from build123d import *

# Parameters (mm, degrees)
SKETCH_1_W      = 53
SKETCH_1_H      = 53
EXTRUDE_1_DEPTH = 10
SKETCH_2_R      = 3


with BuildPart() as part:
    # 草图1 → 凸台-拉伸1 (new body)
    with BuildSketch(Plane.XY):
        with Locations((26.5, 26.5)):
            Rectangle(SKETCH_1_W, SKETCH_1_H)
    extrude(amount=EXTRUDE_1_DEPTH)

    # 扫描1: sweep along a path in 草图4
    with BuildLine(Plane(origin=(0, 0, 0), x_dir=(0, 0, -1), z_dir=(1, 0, 0))) as sweep_1_path:
        Line((-5, 0), (-5, -17))
        Line((-5, -17), (191, -17))
    # 草图2 → 扫描1 (sweep)
    with BuildSketch(Plane(origin=(0, 0, 0), x_dir=(1, 0, 0), z_dir=(0, 1, 0))):
        with Locations((12, -5)):
            Circle(SKETCH_2_R)
    sweep(path=sweep_1_path.line, transition=Transition.RIGHT)


solid = part.part
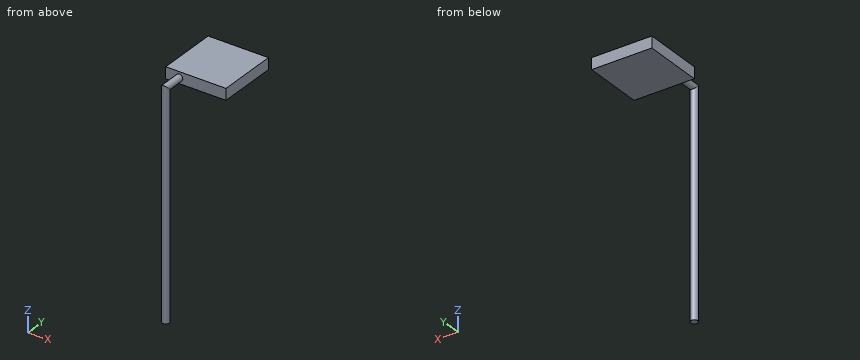
Verification items for the finished model (mm, model axes). Coordinates: 2 decimals unless noted, no trailing zeros. Loops run counter-clockwise (first coordinate to the right, second up) from the corner with the lowest first, then second, coordinate; pieces in that order, holes last. Notation, with made-up numbers: (45, 57.5) -> (54, 57.5) arc R24 ccw to (54, 93.5) -> close; hole circle Ø4 at (56.25, 59). An arc over 180 degrees is marked (long way). Answer as a JSON object with one key per item and string values. Group by question number.
Item 1: Depth check by flat-ended pin: pin 1 (1 mm diameter, centred on x = 11.5, y = 39.5, fed in from -Z); pin 2 (1.5 mm diameter, centred on x = 11, z = -54, fed in from +Y); pin 3 (5 mm diameter, centred on x = 32.5, z = 5, fed in from -Y). Enter the tip coordinate at first touch or a pass-through.
Item 2: Sectioned sample at B-B on z = 5. Record the boundary of the cut face in (x, y).
Item 3: Sectioned sample at A-A on x = 12. Record the boundary of the cut face in (y, z).
Item 4: Sectioned sample at D-D on z = -178. Record the boundary of the cut face in (x, y).
Item 5: Sectioned sample at C-C on y = 31.5. Record the boundary of the cut face in (x, z).
Item 6: Scan lines: probe 1 along Z at (x, y) = (30.5, 21.5); probe 2 along Y at (x, z) = (10.5, -142.5); probe 3 along Z at (x, y) = (13.5, -14). Record each from-to range of solid material in increasing order.
Evaluation:
{
 "1": {"pin 1": "stops at z = 0", "pin 2": "stops at y = -14.01", "pin 3": "stops at y = 0"},
 "2": {"outline": "(0, 0) -> (9, 0) -> (9, -17) arc R3 ccw to (15, -17) -> (15, 0) -> (53, 0) -> (53, 53) -> (0, 53) -> close"},
 "3": {"outline": "(-20, -191) -> (-14, -191) -> (-14, 2) -> (0, 2) -> (0, 0) -> (53, 0) -> (53, 10) -> (0, 10) -> (0, 8) -> (-20, 8) -> close"},
 "4": {"outline": "circle Ø6 at (12, -17)"},
 "5": {"outline": "(0, 0) -> (53, 0) -> (53, 10) -> (0, 10) -> close"},
 "6": {"probe 1": "z = 0 to 10", "probe 2": "y = -19.6 to -14.4", "probe 3": "z = 2.4 to 7.6"}
}
